Check sheet for the modelled part. Datum: model origin and axes. Units: mm. A direction names the side the tool comes from. Coordinates: 2 decimals unless noted, no trailing zeros. Loops run counter-clockwise (first coordinate to the right, second up) from the corner with the lowest first, then second, coordinate; pieces in that order, holes last. Notation, with made-up numbers: (55.25, 76) -> (81.25, 76) arc R29 cw to (81.25, 104) -> close; hole circle Ø1 at (31, 0). An arc over 180 degrees is marked (long way). Use CSV: the item, a comma, the result in double quotes. Start each with the question number.
1. Set-up check for faces 4 (the face through (8.17, -10.01, 31.8)), 5 (the face through (6.87, 15.11, 7.86)): record each of +Z, -Z, +X, -X, +Y, -Y from which the full face is reachable in a straight line by a thin tool's end or side.
2. Gauge pin test, flat ends, axial feed: pin 1 (1 mm diameter, centred on x = 1.5, z = -18.5, fed in from +Y); pin 2 (20.5 mm diameter, centred on y = 0, z = 0, fed in from +X); pin 3 (1 mm diameter, centred on x = 2, z = -21.5, fed in from -Y); pin 4 (5 mm diameter, centred on x = 7, z = 0.5, fed in from +Y). Record the tip position at first contact, or that the pin passes through.
3. Sectioned sample at D-D, the plane x = 8. Record the cut outline in (y, z) (1 decimal).
4. Sectioned sample at A-A, the plane y = 0. Record the cut outline in (x, z), and give its area (3 significant figures).
5. Sectioned sample at C-C, the plane x = 12.25. Record the cut outline in (y, z) (1 decimal).
6. Release check for a two-part mould opening along Z. For faces 1 (the face through (13.564, 13, -31)), 2 (the face through (7.406, 21.228, -27.685)), 3 (the face through (1.76, 22.84, -1.35)) record: pulls with the +Z half, pulls with the -Z half, needs draft (parallel to the pull), parting line crosses it, or undercut.
7. Thickness scan on L1, parallel to Y at x = 1.3, z = 0; L2, parallel to Y at x = 8, z = -5.5; L3, parallel to Z at x = 12, y = 1. Record the ranges inside material, lowest first.
8. Sectioned sample at B-B, the plane z = 0. Count the separate pieces of the cut face and the enclosed holes in it, and give its area (3 significant figures).
```python
from build123d import *

# Parameters (mm, degrees)
SKETCH2_R          = 3.4925
CUT_EXTRUDE1_DEPTH = 52.167986429


with BuildPart() as part:
    # Sketch1 → Revolve1 (revolve)
    with BuildSketch(Plane.XY, mode=Mode.PRIVATE) as revolve1_sk:
        with BuildLine():
            Line((0.155348807, 33.477735982), (1.843834582, 18.161535982))
            ThreePointArc((1.843834582, 18.161535982), (2.258790389, 17.35475119), (3.106186901, 17.0307))
            Line((3.106186901, 17.0307), (10.5283, 17.0307))
            Line((10.5283, 17.0307), (3.88013628, 18.704834032))
            ThreePointArc((3.88013628, 18.704834032), (3.491808651, 18.943062367), (3.308801824, 19.360266859))
            Line((3.308801824, 19.360266859), (1.861135478, 32.492001589))
            ThreePointArc((1.861135478, 32.492001589), (2.050977583, 33.083937907), (2.618546869, 33.3375))
            Line((2.618546869, 33.3375), (13.5636, 33.3375))
            Line((13.5636, 33.3375), (13.5636, 34.8869))
            Line((13.5636, 34.8869), (1.417701126, 34.8869))
            ThreePointArc((1.417701126, 34.8869), (0.471752315, 34.464296512), (0.155348807, 33.477735982))
        make_face()
    revolve(revolve1_sk.sketch.rotate(Axis((-1000.538686221, 0, 0), (1, 0, 0)), 90), axis=Axis((-1000.538686221, 0, 0), (1, 0, 0)))

    # Sketch2 → Cut-Extrude1 (cut, through all)
    with BuildSketch(Plane(origin=(0, 0, 0), x_dir=(0, 0, -1), z_dir=(1, 0, 0))):
        with Locations(Location((0, -26.0604, 0), (0, 0, 315.343502334))):
            Circle(SKETCH2_R)
        with Locations(Location((0, 26.0604, 0), (0, 0, 315.324132172))):
            Circle(SKETCH2_R)
        with Locations(Location((25.4, 0, 0), (0, 0, 314.727093361))):
            Circle(SKETCH2_R)
    extrude(amount=CUT_EXTRUDE1_DEPTH, mode=Mode.SUBTRACT)


solid = part.part
```
Completed:
1,face 4,"+X"
1,face 5,"+X, -X"
2,pin 1,"y = 29.88"
2,pin 2,"through"
2,pin 3,"y = -27.86"
2,pin 4,"y = 34.89"
3,outline,"circle Ø69.8 at (0, 0); circle Ø35.3 at (0, 0); hole circle Ø66.7 at (0, 0); hole circle Ø34.1 at (0, 0)"
4,outline,"(0.16, -33.48) arc R1.27 ccw to (1.42, -34.89) -> (13.56, -34.89) -> (13.56, -33.34) -> (2.62, -33.34) arc R0.76 cw to (1.86, -32.49) -> (2.26, -28.89) -> (0.66, -28.89) -> close; (0.16, 33.48) -> (1.84, 18.16) arc R1.27 ccw to (3.11, 17.03) -> (10.53, 17.03) -> (3.88, 18.7) arc R0.76 cw to (3.31, 19.36) -> (1.86, 32.49) arc R0.76 cw to (2.62, 33.34) -> (13.56, 33.34) -> (13.56, 34.89) -> (1.42, 34.89) arc R1.27 ccw to start; (1.43, -21.91) -> (3.03, -21.91) -> (3.31, -19.36) arc R0.76 cw to (3.88, -18.7) -> (10.53, -17.03) -> (3.11, -17.03) arc R1.27 ccw to (1.84, -18.16) -> close"
4,area,"94.3 mm²"
5,outline,"circle Ø69.8 at (0, 0); hole circle Ø66.7 at (0, 0)"
6,face 1,"needs draft"
6,face 2,"parting line crosses it"
6,face 3,"undercut"
7,L1,"-34.88 to -29.55, 29.55 to 34.88"
7,L2,"-34.45 to -32.88, -16.79 to -16.12, 16.12 to 16.79, 32.88 to 34.45"
7,L3,"-34.87 to -33.32, 33.32 to 34.87"
8,separate pieces,"4"
8,enclosed holes,"0"
8,area,"83.1 mm²"
